```python
from build123d import *

# Parameters (mm, degrees)
EXTRUDE_1_DEPTH     = 6
SKETCH_2_R          = 2
CUT_EXTRUDE_1_DEPTH = 6
SKETCH_3_R          = 5.75
EXTRUDE_2_DEPTH     = 12
SKETCH_4_R          = 1
CUT_EXTRUDE_2_DEPTH = 12


with BuildPart() as part:
    # 草图1 → 凸台-拉伸1 (new body)
    with BuildSketch(Plane(origin=(0, 0, 0), x_dir=(1, 0, 0), z_dir=(0, 1, 0))):
        Polygon((5.280239472, 4.488203551), (-1.246778557, 6.816923297), (-6.527018029, 2.328719745), (-5.280239472, -4.488203551), (1.246778557, -6.816923297), (6.527018029, -2.328719745), align=None)
    extrude(amount=EXTRUDE_1_DEPTH)

    # 草图2 → 切除-拉伸1 (cut)
    with BuildSketch(Plane(origin=(0, 6, 0), x_dir=(1, 0, 0), z_dir=(0, 1, 0))):
        with Locations(Location((0, 0, 0), (0, 0, 270))):
            Circle(SKETCH_2_R)
    extrude(amount=-CUT_EXTRUDE_1_DEPTH, mode=Mode.SUBTRACT)

    # 草图3 → 凸台-拉伸2 (add)
    with BuildSketch(Plane(origin=(0, 6, 0), x_dir=(1, 0, 0), z_dir=(0, 1, 0))):
        with Locations(Location((0, 0, 0), (0, 0, 270))):
            Circle(SKETCH_3_R)
    extrude(amount=EXTRUDE_2_DEPTH)

    # 草图4 → 切除-拉伸2 (cut)
    with BuildSketch(Plane(origin=(0, 18, 0), x_dir=(1, 0, 0), z_dir=(0, 1, 0))):
        with Locations(Location((0, 0, 0), (0, 0, 270))):
            Circle(SKETCH_4_R)
    extrude(amount=-CUT_EXTRUDE_2_DEPTH, mode=Mode.SUBTRACT)


solid = part.part
```
The model under review builds one solid part; all positions refer to its coordinate system, in mm. A direction names the side the tool comes from. Coordinates: 2 decimals unless noted, no trailing zeros. Write each loop counter-clockwise with the first axis right and the second up, starting at its lowest first coordinate (ties: lowest second). Pieces come first, ordered by that corner, then holes. Notation, with made-up numbers: (58, 14.25) -> (92, 14.25) arc R16 ccw to (92, 30.25) -> close; hole circle Ø10 at (87, -16). An arc over 180 degrees is marked (long way). One line per item, written item: value. Start each with the question number.
Q1. Clearance check with flat-ended pins moving along their axes: P1, Ø6, axis at y = 3.5, z = -0.5, coming from the +X side; P2, Ø2.5, axis at x = 0, z = 0, coming from the -Y side; P3, Ø6, axis at y = 14.5, z = 0, coming from the -X side. State where each tip first meets the part, or that it passes through.
Q2. Add section D-D, the plane z = -5.5. Give the boundary of the cut face in (x, y), then the cut area to 3 significant figures.
Q3. For faces 5 (the face through (-1, 6, 1)), 6 (the face through (4.85, 11.92, 3.09)), 7 (the face through (-5.912, 2.958, 1.032)), list the 3-axis set-ups (+Z, -Z, +X, -X, +Y, -Y) from which the entire face can be reached by the end or side of a thin tool; tool diameter is ignored.
Q4. The part is to be moulded in two halves that separate along Z. For faces 1 (the face through (-2.062, 2.958, 5.636)), 2 (the face through (6, 6, 1)), 3 (the face through (-3.85, 2.958, -4.604)), 4 (the face through (-2, 3, 0)), say which applies: +Z half, -Z half, draft (parallel to the pull), parting line (faces both ways), or undercut.
Q5. To check wall thickness, follow probe 1 along X at (y, z) = (12.75, 0); probe 2 along Y at (x, z) = (0.25, -6); probe 3 along X at (y, z) = (2.7, 0). State the ranges of each line that lie inside material, in increasing order.
Q6. Add section B-B, the plane z = 0.25. Give the boundary of the cut face in (x, y), then the cut area to 3 significant figures.
Q7. Add section A-A, the plane y = 1. Give the boundary of the cut face in (x, z).
Q8. Add section C-C, the plane x = 0. Give the boundary of the cut face in (y, z).
Response:
1. P1: x = 6.53
1. P2: y = 6
1. P3: x = -5.75
2. outline: (-2.8, 0) -> (2.44, 0) -> (2.44, 6) -> (1.68, 6) -> (1.68, 18) -> (-1.68, 18) -> (-1.68, 6) -> (-2.8, 6) -> close
2. area: 71.7 mm²
3. face 5: -Y
3. face 6: +Y
3. face 7: +Z, -X, +Y, -Y
4. face 1: +Z half
4. face 2: draft
4. face 3: -Z half
4. face 4: undercut
5. probe 1: -5.75 to -1, 1 to 5.75
5. probe 2: 0 to 6
5. probe 3: -6.1 to -2, 2 to 6.1
6. outline: (-6.06, 0) -> (-1.98, 0) -> (-1.98, 6) -> (-0.97, 6) -> (-0.97, 18) -> (-5.74, 18) -> (-5.74, 6) -> (-6.06, 6) -> close; (0.97, 6) -> (1.98, 6) -> (1.98, 0) -> (6.15, 0) -> (6.15, 6) -> (5.74, 6) -> (5.74, 18) -> (0.97, 18) -> close
6. area: 164 mm²
7. outline: (-6.53, -2.33) -> (-1.25, -6.82) -> (5.28, -4.49) -> (6.53, 2.33) -> (1.25, 6.82) -> (-5.28, 4.49) -> close; hole circle Ø4 at (0, 0)
8. outline: (0, -6.37) -> (6, -6.37) -> (6, -5.75) -> (18, -5.75) -> (18, -1) -> (6, -1) -> (6, -2) -> (0, -2) -> close; (0, 2) -> (6, 2) -> (6, 1) -> (18, 1) -> (18, 5.75) -> (6, 5.75) -> (6, 6.37) -> (0, 6.37) -> close
